Verification items for the finished model (mm, model axes). Face numbers are marked on the shaded views. Give positions to 0.01 mm unless a question says otherwise; leave off trailing zeros. Loops run counter-clockwise (first coordinate to the right, second up) from the corner with the lowest first, then second, coordinate; pieces in that order, holes last. Notation, with made-up numbers: M 78,-34.75 L 97,-34.75 A17 ccw 97,-20.75 Z; hole C -25,40 d3. An arc over 180 degrees is marked long. Answer in a Markdown table with one row per item.
```python
from build123d import *

# Parameters (mm, degrees)
ESQUISSE1_R        = 16
ESQUISSE1_R_2      = 3.25
ESQUISSE1_R_3      = 1.5
BOSS_EXTRU_1_DEPTH = 3


with BuildPart() as part:
    # Esquisse1 → Boss.-Extru.1 (new body)
    with BuildSketch(Plane.XY):
        Circle(ESQUISSE1_R)
        with Locations((5.508433282, -9.231449657)):
            Circle(ESQUISSE1_R_2, mode=Mode.SUBTRACT)
        with Locations((-10.748886558, -0.154718329)):
            Circle(ESQUISSE1_R_2, mode=Mode.SUBTRACT)
        with Locations((5.240453276, 9.386167986)):
            Circle(ESQUISSE1_R_2, mode=Mode.SUBTRACT)
        with Locations((1.70619409, 3.05596167)):
            Circle(ESQUISSE1_R_3, mode=Mode.SUBTRACT)
        with Locations((-1.70619409, -3.05596167)):
            Circle(ESQUISSE1_R_3, mode=Mode.SUBTRACT)
        with BuildLine():
            ThreePointArc((-1.54267531, 3.141679947), (0.121871006, 0.218282976), (3.483906341, 0.335256035))
            ThreePointArc((3.483906341, 0.335256035), (3.05596167, -1.70619409), (1.54267531, -3.141679947))
            ThreePointArc((1.54267531, -3.141679947), (-0.121871006, -0.218282976), (-3.483906341, -0.335256035))
            ThreePointArc((-3.483906341, -0.335256035), (-3.05596167, 1.70619409), (-1.54267531, 3.141679947))
        make_face(mode=Mode.SUBTRACT)
    extrude(amount=BOSS_EXTRU_1_DEPTH)


solid = part.part
```
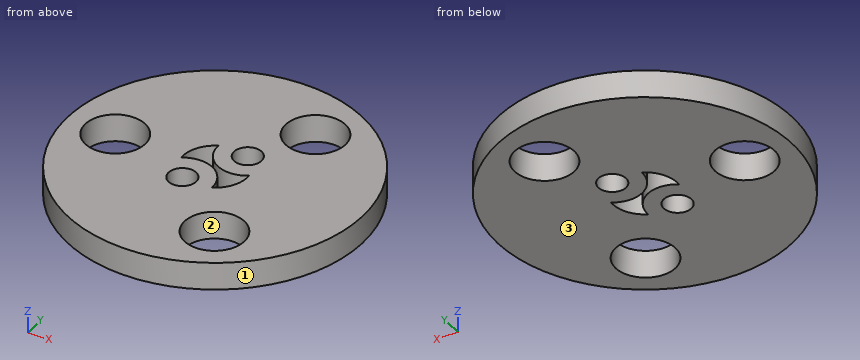
Item 1: Sectioned sample at C-C (y = -12). Record the cut outline in (x, z).
Reported:
| item | result |
|---|---|
| outline | M -10.58,0 L 3.81,0 L 3.81,3 L -10.58,3 Z; M 7.21,0 L 10.58,0 L 10.58,3 L 7.21,3 Z |
Item 2: Sectioned sample at A-A (y = -8). Record the cut outline in (x, z), and give its area (3 significant figures).
Reported:
| item | result |
|---|---|
| outline | M -13.86,0 L 2.5,0 L 2.5,3 L -13.86,3 Z; M 8.52,0 L 13.86,0 L 13.86,3 L 8.52,3 Z |
| area | 65.1 mm^2 |
Item 3: Release check for a two-part mould opening along X. For the marked faces 1, 2 and 3 record: released by +X, released by -X, zero draft, split by the parting line, or undercut.
Reported:
| item | result |
|---|---|
| face 1 | split by the parting line |
| face 2 | undercut |
| face 3 | zero draft |
Item 4: Scan lines: L1, parallel to X at y = 0.5, z = 0.8; L2, parallel to Y at x = 7, z = 0.85; L3, parallel to Y at x = 1, z = 1.75. Record each from-to range of solid material in increasing order. Write a range as [from, to].
Reported:
| item | result |
|---|---|
| L1 | x = [-15.99, -13.93], [-7.57, -3.46], [-0.3, 15.99] |
| L2 | y = [-14.39, -12.12], [-6.34, 6.65], [12.12, 14.39] |
| L3 | y = [-15.97, -1.26], [-0.12, 1.73], [4.38, 15.97] |
Item 5: Sectioned sample at D-D (x = -4). Record the cut outline in (y, z), and give its area (3 significant figures).
Reported:
| item | result |
|---|---|
| outline | M -15.49,0 L 15.49,0 L 15.49,3 L -15.49,3 Z |
| area | 93.0 mm^2 |
Item 6: Sectioned sample at B-B (z = 1.45). Record the cut outline in (x, y).
Reported:
| item | result |
|---|---|
| outline | C 0,0 d32; hole C -10.75,-0.15 d6.5; hole M -3.48,-0.34 A3.25 cw 1.54,-3.14 A3.5 ccw 3.48,0.34 A3.25 cw -1.54,3.14 A3.5 ccw Z; hole C -1.71,-3.06 d3; hole C 1.71,3.06 d3; hole C 5.24,9.39 d6.5; hole C 5.51,-9.23 d6.5 |
Item 7: Go/stop test with a flat-tipped pin: pin 1 (6 mm diameter, centred on x = 5.24, y = 9.39, fed in from -Z). Record where the tip stops, or that it passes through.
Reported:
| item | result |
|---|---|
| pin 1 | passes through |
